Could you check a few things on this model? Use its own coordinates, in mm. A direction names the side the tool comes from. Give positions to 0.01 mm unless a question says otherwise; leave off trailing zeros. Order: outer loops, then holes, each group sorted by start corner. A loop starts at its lowest first (then second) coordinate and runs counter-clockwise, first axis right, second up. Notation, with made-up numbers: (40, 75) -> (52, 75) arc R17 ccw to (52, 100) -> close; hole circle Ø3 at (-1, 53.5). An arc over 180 degrees is marked (long way). Answer as CSV lines item,"result". Start each with the question number.
(1) We'd pull the mould along Z, two halves only. Please class faces 1 (the face through (-14, 6.5, -13.8)), 2 (the face through (-9, 15, -12)), 3 (the face through (27.65, 2.028, -9.904)): released by +Z, released by -Z, zero draft, split by the parting line, or undercut.
(2) I want a section at A-A (z = 0). Please give me the cut outline in (x, y).
(3) I want a section at D-D (y = 5.5). Please give me the cut outline in (x, z), plus the area to 3 significant figures.
(4) I want a section at B-B (y = 1.75). Please give me the cut outline in (x, z), plus the area to 3 significant figures.
(5) On a 3-axis mill with a long thin cutter (end or side, diameter ignored), from which of +Z, -Z, +X, -X, +Y, -Y can I reach the whole of each face in a straight line? I mean faces 4 (the face through (-27.65, 2.028, -9.904)), 5 (the face through (0, 3, -11)), 6 (the face through (-11.5, 14, -10)). Say none if no direction works.
(6) I want a section at C-C (x = -21.5). Please give me the cut outline in (y, z), plus the area to 3 significant figures.
(7) Will these pins go through, and if not, where does the flat tip stop? pin 1 Ø1.5 at (x, z) = (18.5, 23.5) entering from +Y; pin 2 Ø1.5 at (x, y) = (-13, 9.5) entering from -Z; pin 3 Ø3.5 at (x, y) = (6.5, 4.5) entering from -Z; pin 4 Ø5 at (y, z) = (13, -11) entering from -X.
(8) I need wall thicknesses on L1, parallel to X at y = 0.9, z = 0; L2, parallel to Y at x = -20, z = -15; L3, parallel to X at y = 1.25, z = 25.5. Which ranges of each line are inside material? Lowest first, please.
```python
from build123d import *

# Parameters (mm, degrees)
SKETCH1_R           = 34.25
SKETCH1_R_2         = 30.25
BOSS_EXTRUDE1_DEPTH = 4
BOSS_EXTRUDE2_START = -11.5
BOSS_EXTRUDE2_DEPTH = 6
BOSS_EXTRUDE3_START = 4
BOSS_EXTRUDE3_DEPTH = 4
CHAMFER1_SIZE       = 5
FILLET1_R           = 5
CUT_EXTRUDE2_REACH  = 58.809
SKETCH6_R           = 1.65


with BuildPart() as part:
    # Sketch1 → Boss-Extrude1 (new body)
    with BuildSketch(Plane(origin=(0, 0, 0), x_dir=(1, 0, 0), z_dir=(0, 1, 0))):
        with Locations(Location((0, 0, 0), (0, 0, 270))):
            Circle(SKETCH1_R)
        with Locations(Location((0, 0, 0), (0, 0, 270))):
            Circle(SKETCH1_R_2, mode=Mode.SUBTRACT)
    extrude(amount=BOSS_EXTRUDE1_DEPTH)



with BuildPart() as body_2:
    # Sketch2 → Boss-Extrude2 (new body)
    with BuildSketch(Plane(origin=(0, 0, 0), x_dir=(0, 0, -1), z_dir=(1, 0, 0)).offset(BOSS_EXTRUDE2_START)):
        Polygon((3.97918472, 15.949747468), (11, 8.928932188), (11, 4), (16, 4), (16, 11), (7.514718626, 19.485281374), align=None)
    extrude(amount=BOSS_EXTRUDE2_DEPTH)


with BuildPart() as part_1:
    add(part.part)

    add(body_2.part)  # Boss-Extrude3 merges body 2
    # Sketch5 → Boss-Extrude3 (add)
    with BuildSketch(Plane.XZ.offset(-4).offset(BOSS_EXTRUDE3_START)):
        with BuildLine():
            Line((28.179114606, -11), (-28.179114606, -11))
            ThreePointArc((-28.179114606, -11), (-27.041474823, -13.558065475), (-25.672212604, -16))
            Line((-25.672212604, -16), (25.672212604, -16))
            ThreePointArc((25.672212604, -16), (27.041474823, -13.558065475), (28.179114606, -11))
        make_face()
    extrude(amount=-BOSS_EXTRUDE3_DEPTH)

    # Chamfer1
    # the kernel refuses this chamfer: 5 mm, written as the material it adds along each edge
    with BuildSketch(Plane(origin=(-11.5, 4, 1.85841494), x_dir=(-0.9996219169112968, -0.027495876610586403, 0), z_dir=(0, 0, -1))) as chamfer1_piece_1_section:
        Polygon((CHAMFER1_SIZE * 0.999621916911, CHAMFER1_SIZE * 0.0274958766106), (-CHAMFER1_SIZE * 0.0274958766106, CHAMFER1_SIZE * 0.999621916911), (0, 0), align=None)
    chamfer1_piece_1 = extrude(amount=17.85841494, mode=Mode.PRIVATE)
    chamfer1_piece_1 = split(chamfer1_piece_1, bisect_by=Plane(origin=(-11.354428767, 9.056622431, -11), z_dir=(0, 0, 1)), keep=Keep.TOP, mode=Mode.PRIVATE)
    chamfer1_piece_1 = split(chamfer1_piece_1, bisect_by=Plane(origin=(-11.354428767, 9.02469987, -10.904232318), z_dir=(0, 0.7071067811865489, -0.7071067811865462)), keep=Keep.TOP, mode=Mode.PRIVATE)
    add(chamfer1_piece_1)
    with BuildSketch(Plane(origin=(-11.5, 4, -11), x_dir=(-0.9996219169112968, -0.027495876610586924, 0), z_dir=(0, 0, -1))) as chamfer1_piece_2_section:
        Polygon((CHAMFER1_SIZE * 0.999621916911, CHAMFER1_SIZE * 0.0274958766106), (-CHAMFER1_SIZE * 0.0274958766106, CHAMFER1_SIZE * 0.999621916911), (0, 0), align=None)
    chamfer1_piece_2 = extrude(amount=5, mode=Mode.PRIVATE)
    chamfer1_piece_2 = split(chamfer1_piece_2, bisect_by=Plane(origin=(-13.406884942, 6.106803662, -13.822128526), z_dir=(0, -0.7071067811865489, 0.7071067811865462)), keep=Keep.TOP, mode=Mode.PRIVATE)
    add(chamfer1_piece_2)
    with BuildSketch(Plane(origin=(-11.5, 4, -11), x_dir=(-0.9996219169112968, -0.027495876610586924, 0), z_dir=(0, 0, -1))) as chamfer1_piece_3_section:
        Polygon((CHAMFER1_SIZE * 0.999621916911, CHAMFER1_SIZE * 0.0274958766106), (-CHAMFER1_SIZE * 0.0274958766106, CHAMFER1_SIZE * 0.999621916911), (0, 0), align=None)
    chamfer1_piece_3 = extrude(amount=5, mode=Mode.PRIVATE)
    chamfer1_piece_3 = split(chamfer1_piece_3, bisect_by=Plane(origin=(-12.657418843, 5.909631949, -14.019300239), z_dir=(0, 0.7071067811865489, -0.7071067811865462)), keep=Keep.TOP, mode=Mode.PRIVATE)
    add(chamfer1_piece_3)
    with BuildSketch(Plane(origin=(-5.5, 4, 1.85841494), x_dir=(0.9996219169112968, -0.027495876610586403, 0), z_dir=(0, 0, -1))) as chamfer1_piece_4_section:
        Polygon((CHAMFER1_SIZE * 0.999621916911, -CHAMFER1_SIZE * 0.0274958766106), (-CHAMFER1_SIZE * 0.0274958766106, -CHAMFER1_SIZE * 0.999621916911), (0, 0), align=None)
    chamfer1_piece_4 = extrude(amount=17.85841494, mode=Mode.PRIVATE)
    chamfer1_piece_4 = split(chamfer1_piece_4, bisect_by=Plane(origin=(-5.645571233, 9.056622431, -11), z_dir=(0, 0, 1)), keep=Keep.TOP, mode=Mode.PRIVATE)
    chamfer1_piece_4 = split(chamfer1_piece_4, bisect_by=Plane(origin=(-5.645571233, 9.02469987, -10.904232318), z_dir=(0, 0.7071067811865489, -0.7071067811865462)), keep=Keep.TOP, mode=Mode.PRIVATE)
    add(chamfer1_piece_4)
    with BuildSketch(Plane(origin=(-5.5, 4, -11), x_dir=(0.9996219169112968, -0.027495876610586924, 0), z_dir=(0, 0, -1))) as chamfer1_piece_5_section:
        Polygon((CHAMFER1_SIZE * 0.999621916911, -CHAMFER1_SIZE * 0.0274958766106), (-CHAMFER1_SIZE * 0.0274958766106, -CHAMFER1_SIZE * 0.999621916911), (0, 0), align=None)
    chamfer1_piece_5 = extrude(amount=5, mode=Mode.PRIVATE)
    chamfer1_piece_5 = split(chamfer1_piece_5, bisect_by=Plane(origin=(-3.593115058, 6.106803662, -13.822128526), z_dir=(0, -0.7071067811865489, 0.7071067811865462)), keep=Keep.TOP, mode=Mode.PRIVATE)
    add(chamfer1_piece_5)
    with BuildSketch(Plane(origin=(-5.5, 4, -11), x_dir=(0.9996219169112968, -0.027495876610586924, 0), z_dir=(0, 0, -1))) as chamfer1_piece_6_section:
        Polygon((CHAMFER1_SIZE * 0.999621916911, -CHAMFER1_SIZE * 0.0274958766106), (-CHAMFER1_SIZE * 0.0274958766106, -CHAMFER1_SIZE * 0.999621916911), (0, 0), align=None)
    chamfer1_piece_6 = extrude(amount=5, mode=Mode.PRIVATE)
    chamfer1_piece_6 = split(chamfer1_piece_6, bisect_by=Plane(origin=(-4.342581157, 5.909631949, -14.019300239), z_dir=(0, 0.7071067811865489, -0.7071067811865462)), keep=Keep.TOP, mode=Mode.PRIVATE)
    add(chamfer1_piece_6)

    # Fillet1
    fillet1_edges = [part_1.edges().sort_by_distance(p)[0] for p in [
        (-25.672212604, 2, -16),
        (-28.179114606, 2, -11),
        (28.179114606, 2, -11),
        (25.672212604, 2, -16),
    ]]
    fillet(fillet1_edges, radius=FILLET1_R)

    # Sketch6 → Cut-Extrude2 (cut, up to next)
    with BuildSketch(Plane(origin=(0, 9.964466094, -9.964466094), x_dir=(1, 0, 0), z_dir=(0, -0.7071067811865487, 0.7071067811865464)), mode=Mode.PRIVATE) as cut_extrude2_sk1:
        with Locations(Location((-8.5, 4.535533906, 0), (0, 0, 270))):
            Circle(SKETCH6_R)
    cut_extrude2_tool1 = extrude(cut_extrude2_sk1.sketch, amount=-CUT_EXTRUDE2_REACH, mode=Mode.PRIVATE) & part_1.part
    add(cut_extrude2_tool1.solids().sort_by_distance((-8.5, 13.171573, -6.757359))[0], mode=Mode.SUBTRACT)


solid = part_1.part
```
Final values:
1,face 1,"zero draft"
1,face 2,"released by -Z"
1,face 3,"undercut"
2,outline,"(-34.25, 0) -> (-30.25, 0) -> (-30.25, 4) -> (-34.25, 4) -> close; (30.25, 0) -> (34.25, 0) -> (34.25, 4) -> (30.25, 4) -> close"
3,outline,"(-15, -16.1) arc R5 cw to (-14.02, -16) -> (-2, -16) -> (-2, -11) -> (-15, -11) -> close"
3,area,"65.0 mm²"
4,outline,"circle Ø68.5 at (0, 0); hole (-29.38, -7.19) arc R5 ccw to (-24.53, -11) -> (24.53, -11) arc R5 ccw to (29.38, -7.19) arc R30.25 ccw (long way) to start; hole (-16.8, -25.16) arc R30.25 ccw to (16.8, -25.16) arc R5 ccw to (14.02, -16) -> (-14.02, -16) arc R5 ccw to start"
4,area,"1,150 mm²"
5,face 4,"+Y, -Y"
5,face 5,"-Y"
5,face 6,"+Z, -Z, -X, +Y"
6,outline,"(0, -26.66) -> (4, -26.66) -> (4, -11) -> (0, -11) -> close; (0, 21.28) -> (4, 21.28) -> (4, 26.66) -> (0, 26.66) -> close"
6,area,"84.2 mm²"
7,pin 1,"y = 4"
7,pin 2,"through"
7,pin 3,"z = -33.91"
7,pin 4,"x = -11.5"
8,L1,"-34.25 to -30.25, 30.25 to 34.25"
8,L2,"0 to 4"
8,L3,"-22.87 to -16.27, 16.27 to 22.87"
